The model under review builds one solid part; all positions refer to its coordinate system, in mm. Face numbers are marked on the shaded views. Coordinates: 2 decimals unless noted, no trailing zeros. Write each loop counter-clockwise with the first axis right and the second up, starting at its lowest first coordinate (ties: lowest second). Pieces come first, ordered by that corner, then holes. Notation, with made-up numbers: (7, 48) - (36, 48) arc R24 cw to (36, 74) - close; hole circle Ø8 at (11, 63.25). An arc over 180 degrees is marked (long way). Answer as CSV lines item,"result". Start each with the question number.
```python
from build123d import *

# Parameters (mm, degrees)
SKETCH_2_W          = 20
SKETCH_2_H          = 25
SKETCH_2_R          = 7.675
EXTRUDE_1_DEPTH     = 100
SKETCH_3_R          = 2.15
SKETCH_3_R_2        = 4.15
CUT_EXTRUDE_2_DEPTH = 104.561575886
CHAMFER_1_SIZE      = 1
CHAMFER_2_SIZE      = 1


with BuildPart() as part:
    # Sketch 2 → Extrude 1 (new body)
    with BuildSketch(Plane.XY):
        Rectangle(SKETCH_2_W, SKETCH_2_H)
        Circle(SKETCH_2_R, mode=Mode.SUBTRACT)
    extrude(amount=-EXTRUDE_1_DEPTH)

    # Sketch 3 → Cut-Extrude 2 (cut, through all)
    with BuildSketch(Plane(origin=(0, 12.5, 0), x_dir=(1, 0, 0), z_dir=(0, 1, 0))):
        with Locations(Location((0, 75, 0), (0, 0, 270))):
            Circle(SKETCH_3_R)
        with Locations(Location((0, 50, 0), (0, 0, 270))):
            Circle(SKETCH_3_R_2)
        with Locations(Location((0, 90, 0), (0, 0, 270))):
            Circle(SKETCH_3_R)
        with Locations(Location((0, 10, 0), (0, 0, 270))):
            Circle(SKETCH_3_R)
        with Locations(Location((0, 25, 0), (0, 0, 270))):
            Circle(SKETCH_3_R)
    extrude(amount=-CUT_EXTRUDE_2_DEPTH, mode=Mode.SUBTRACT)

    # Chamfer 1
    chamfer_1_edges = [part.edges().sort_by_distance(p)[0] for p in [
        (-7.675, 0, -100),
        (-7.675, 0, 0),
        (-10, 0, -100),
        (0, -12.5, -100),
        (10, 0, -100),
        (0, -12.5, 0),
        (-10, 0, 0),
        (0, 12.5, 0),
        (10, 0, 0),
        (0, 12.5, -100),
    ]]
    chamfer(chamfer_1_edges, length=CHAMFER_1_SIZE)

    # Chamfer 2
    chamfer_2_edges = [part.edges().sort_by_distance(p)[0] for p in [
        (10, 12.5, -50),
        (-10, 12.5, -50),
        (-10, -12.5, -50),
        (10, -12.5, -50),
    ]]
    chamfer(chamfer_2_edges, length=CHAMFER_2_SIZE)


solid = part.part
```
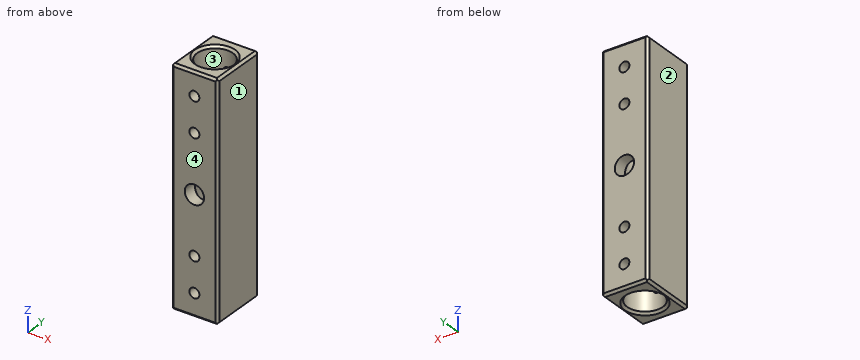
(1) Add section D-D on x = 0. Give the number of separate pieces and of enclosed holes in the cut face, then the cut area to 3 significant figures.
(2) Add section A-A on y = 0. Give the boundary of the cut face in (x, z) (3 decimals), then the cut area to 3 significant figures.
(3) The part is to be moulded in two halves that separate along X. For the marked faces 1, 2, 3 and 4, say which applies: released by +X, released by -X, zero draft, split by the parting line, or undercut.
(4) Add section B-B on z = -59.5. Give the boundary of the cut face in (x, y) (3 decimals).
(5) Wall thickness on line 1 (Z direction, x = 0, y = -10); line 2 (Y direction, x = 0, z = -21.5) (3 decimals); line 3 (X direction, y = -11.2, z = -10): over which ranges is each line inside the solid? List them lowest first.
(6) Add section C-C on z = -25. Give the boundary of the cut face in (x, y) (3 decimals).
Reported:
1,separate pieces,"12"
1,enclosed holes,"0"
1,area,"715 mm²"
2,outline,"(-10, -99) - (-9, -100) - (-8.675, -100) - (-7.675, -99) - (-7.675, -1) - (-8.675, 0) - (-9, 0) - (-10, -1) - close; (7.675, -99) - (8.675, -100) - (9, -100) - (10, -99) - (10, -1) - (9, 0) - (8.675, 0) - (7.675, -1) - close"
2,area,"461 mm²"
3,face 1,"released by +X"
3,face 2,"released by -X"
3,face 3,"undercut"
3,face 4,"zero draft"
4,outline,"(-10, -11.5) - (-9, -12.5) - (9, -12.5) - (10, -11.5) - (10, 11.5) - (9, 12.5) - (-9, 12.5) - (-10, 11.5) - close; hole circle Ø15.35 at (0, 0)"
5,line 1,"-100 to -92.15, -87.85 to -77.15, -72.85 to -54.15, -45.85 to -27.15, -22.85 to -12.15, -7.85 to 0"
5,line 2,"-12.5 to -7.675, 7.675 to 12.5"
5,line 3,"-10 to -2.15, 2.15 to 10"
6,outline,"(-10, -11.5) - (-9, -12.5) - (-2.15, -12.5) - (-2.15, -7.368) arc R7.675 cw to (-2.15, 7.368) - (-2.15, 12.5) - (-9, 12.5) - (-10, 11.5) - close; (2.15, -12.5) - (9, -12.5) - (10, -11.5) - (10, 11.5) - (9, 12.5) - (2.15, 12.5) - (2.15, 7.368) arc R7.675 cw to (2.15, -7.368) - close"
